from build123d import *

# Parameters (mm, degrees)
SKETCH1_W                                      = 104.775
SKETCH1_H                                      = 53.975
BOSS_EXTRUDE1_DEPTH                            = 12.7
SKETCH3_W                                      = 89.916
SKETCH3_H                                      = 31.496
SKETCH3_W_2                                    = 86.36
SKETCH3_H_2                                    = 27.94
CUT_EXTRUDE1_DEPTH                             = 1.905
FILLET1_R                                      = 1.905
SKETCH4_R                                      = 2.159
CUT_EXTRUDE2_DEPTH                             = 61.283209209
SKETCH8_R                                      = 3.6195
CUT_EXTRUDE3_DEPTH                             = 4.572
FILLET2_R                                      = 3.81
SKETCH13_W                                     = 66.04
SKETCH13_H                                     = 12.7
CUT_EXTRUDE4_DEPTH                             = 61.283209209
CBORE_FOR_4_SOCKET_HEAD_CAP_SCREW3_D           = 3.2639
CBORE_FOR_4_SOCKET_HEAD_CAP_SCREW3_CBORE_D     = 5.55752
CBORE_FOR_4_SOCKET_HEAD_CAP_SCREW3_CBORE_DEPTH = 2.8448


with BuildPart() as part:
    # Sketch1 → Boss-Extrude1 (new body)
    with BuildSketch(Plane(origin=(0, 0, 0), x_dir=(1, 0, 0), z_dir=(0, 1, 0))):
        Rectangle(SKETCH1_W, SKETCH1_H)
    extrude(amount=BOSS_EXTRUDE1_DEPTH)

    # Sketch3 → Cut-Extrude1 (cut)
    with BuildSketch(Plane(origin=(0, 12.7, 0), x_dir=(1, 0, 0), z_dir=(0, 1, 0))):
        Rectangle(SKETCH3_W, SKETCH3_H)
        Rectangle(SKETCH3_W_2, SKETCH3_H_2, mode=Mode.SUBTRACT)
    extrude(amount=-CUT_EXTRUDE1_DEPTH, mode=Mode.SUBTRACT)

    # Fillet1
    fillet1_edges = [part.edges().sort_by_distance(p)[0] for p in [
        (43.18, 11.7475, 13.97),
        (-43.18, 11.7475, 13.97),
        (-43.18, 11.7475, -13.97),
        (43.18, 11.7475, -13.97),
    ]]
    fillet(fillet1_edges, radius=FILLET1_R)

    # Sketch4 → Cut-Extrude2 (cut, through all)
    with BuildSketch(Plane.XZ):
        with Locations(Location((-46.99, 21.59, 0), (0, 0, 270))):
            Circle(SKETCH4_R)
        with Locations(Location((46.99, 21.59, 0), (0, 0, 270))):
            Circle(SKETCH4_R)
        with Locations(Location((-46.99, -21.59, 0), (0, 0, 270))):
            Circle(SKETCH4_R)
        with Locations(Location((46.99, -21.59, 0), (0, 0, 270))):
            Circle(SKETCH4_R)
        with Locations(Location((0, 21.59, 0), (0, 0, 270))):
            Circle(SKETCH4_R)
        with Locations(Location((0, -21.59, 0), (0, 0, 270))):
            Circle(SKETCH4_R)
    extrude(amount=-CUT_EXTRUDE2_DEPTH, mode=Mode.SUBTRACT)

    # Sketch8 → Cut-Extrude3 (cut)
    with BuildSketch(Plane.XZ):
        with Locations(Location((-46.99, 21.59, 0), (0, 0, 270))):
            Circle(SKETCH8_R)
        with Locations(Location((0, 21.59, 0), (0, 0, 270))):
            Circle(SKETCH8_R)
        with Locations(Location((46.99, 21.59, 0), (0, 0, 270))):
            Circle(SKETCH8_R)
        with Locations(Location((46.99, -21.59, 0), (0, 0, 270))):
            Circle(SKETCH8_R)
        with Locations(Location((0, -21.59, 0), (0, 0, 270))):
            Circle(SKETCH8_R)
        with Locations(Location((-46.99, -21.59, 0), (0, 0, 270))):
            Circle(SKETCH8_R)
    extrude(amount=-CUT_EXTRUDE3_DEPTH, mode=Mode.SUBTRACT)

    # Fillet2
    fillet2_edges = [part.edges().sort_by_distance(p)[0] for p in [
        (52.3875, 6.35, 26.9875),
        (-52.3875, 6.35, 26.9875),
        (-52.3875, 6.35, -26.9875),
        (52.3875, 6.35, -26.9875),
    ]]
    fillet(fillet2_edges, radius=FILLET2_R)

    # Sketch13 → Cut-Extrude4 (cut, through all)
    with BuildSketch(Plane.XZ):
        Rectangle(SKETCH13_W, SKETCH13_H)
    extrude(amount=-CUT_EXTRUDE4_DEPTH, mode=Mode.SUBTRACT)

    # CBORE for #4 Socket Head Cap Screw3 (through all)
    with Locations(Plane(origin=(0, 12.7, 0), x_dir=(1, 0, 0), z_dir=(0, 1, 0))):
        with Locations((-38.1, 0), (38.1, 0)):
            CounterBoreHole(CBORE_FOR_4_SOCKET_HEAD_CAP_SCREW3_D / 2, CBORE_FOR_4_SOCKET_HEAD_CAP_SCREW3_CBORE_D / 2, CBORE_FOR_4_SOCKET_HEAD_CAP_SCREW3_CBORE_DEPTH)


solid = part.part
Can you work these out from the model? Positions are in its coordinate system, mm. A direction names the side the tool comes from. Coordinates: 2 decimals unless noted, no trailing zeros. Loops run counter-clockwise (first coordinate to the right, second up) from the corner with the lowest first, then second, coordinate; pieces in that order, holes last. Notation, with made-up numbers: M 64,87 L 85,87 A16 ccw 85,103 Z; hole C -30.75,65 d8. An arc over 180 degrees is marked long. Answer as CSV lines item,"result". Start each with the question number.
1. Suppose I cut it at B-B, the plane z = -21.59. List the corners of the cut face in (x, y) for me.
2. For faces 4 (the face through (0, 6, 6.35)), 5 (the face through (-38, 9.855, 2)), 6 (the face through (45, 4.572, -23)), 7 (the face through (-1, 12.7, -18)), which set-ups out of +Z, -Z, +X, -X, +Y, -Y let a thin tool reach every point of the face, with its end or its side?
3. If I drill on probe 1 along X at (y, z) = (1.25, 21.59); probe 2 along Z at (x, y) = (20, 11.75); probe 3 along X at (y, z) = (11, -12), over which ranges is the centre line in solid material (lowest first)? Write a range as [from, to].
4. Suppose I cut it at D-D, the plane x = 38.1. List the corners of the cut face in (y, z) for me (1 decimal), plus the area to 3 significant figures.
5. Suppose I cut it at A-A, the plane y = 11.75. Count the separate pieces of the cut face and the enclosed holes in it, plus the area to 3 significant figures.
6. For pin 1 Ø7 at (x, z) = (-46.99, -21.59) entering from +Y; pin 2 Ø7 at (x, z) = (0, -21.59) entering from -Y; pin 3 Ø4 at (x, z) = (0, 21.59) entering from +Y, each with a flat end and sliding along its axis, tell me the tip position at first contact or that it passes through.
7. Thinking about a two-plate mould opening in Z: for faces 1 (the face through (-33.02, 6, 0)), 2 (the face through (-51.3, 6.44, 25.84)), 3 (the face through (-1, 6, -26.988)), which applies, +Z half, -Z half, draft (parallel to the pull), parting line (faces both ways), or undercut?
Output:
1,outline,"M -52.39,0 L -50.61,0 L -50.61,4.57 L -49.15,4.57 L -49.15,12.7 L -52.39,12.7 Z; M -44.83,4.57 L -43.37,4.57 L -43.37,0 L -3.62,0 L -3.62,4.57 L -2.16,4.57 L -2.16,12.7 L -44.83,12.7 Z; M 2.16,4.57 L 3.62,4.57 L 3.62,0 L 43.37,0 L 43.37,4.57 L 44.83,4.57 L 44.83,12.7 L 2.16,12.7 Z; M 49.15,4.57 L 50.61,4.57 L 50.61,0 L 52.39,0 L 52.39,12.7 L 49.15,12.7 Z"
2,face 4,"+Y, -Y"
2,face 5,"+Y"
2,face 6,"-Y"
2,face 7,"+Z, -Z, +X, -X, +Y"
3,probe 1,"x = [-52.39, -50.61], [-43.37, -3.62], [3.62, 43.37], [50.61, 52.39]"
3,probe 2,"z = [-26.99, -15.75], [-13.97, -6.35], [6.35, 13.97], [15.75, 26.99]"
3,probe 3,"x = [-52.39, -44.96], [-43.18, 43.18], [44.96, 52.39]"
4,outline,"M 0,-27 L 12.7,-27 L 12.7,-15.7 L 10.8,-15.7 L 10.8,-14 L 12.7,-14 L 12.7,-2.8 L 9.9,-2.8 L 9.9,-1.6 L 0,-1.6 Z; M 0,1.6 L 9.9,1.6 L 9.9,2.8 L 12.7,2.8 L 12.7,14 L 10.8,14 L 10.8,15.7 L 12.7,15.7 L 12.7,27 L 0,27 Z"
4,area,"631 mm^2"
5,separate pieces,"2"
5,enclosed holes,"10"
5,area,"4,250 mm^2"
6,pin 1,"stops at y = 12.7"
6,pin 2,"stops at y = 4.57"
6,pin 3,"passes through"
7,face 1,"undercut"
7,face 2,"+Z half"
7,face 3,"-Z half"
